Part print with two shaded views. Sizes in mm from the minimum x, y, z corner. Coordinates: 2 decimals unless noted, no trailing zeros. Loops run counter-clockwise (first coordinate to the right, second up) from the corner with the lowest first, then second, coordinate; pieces in that order, holes last.
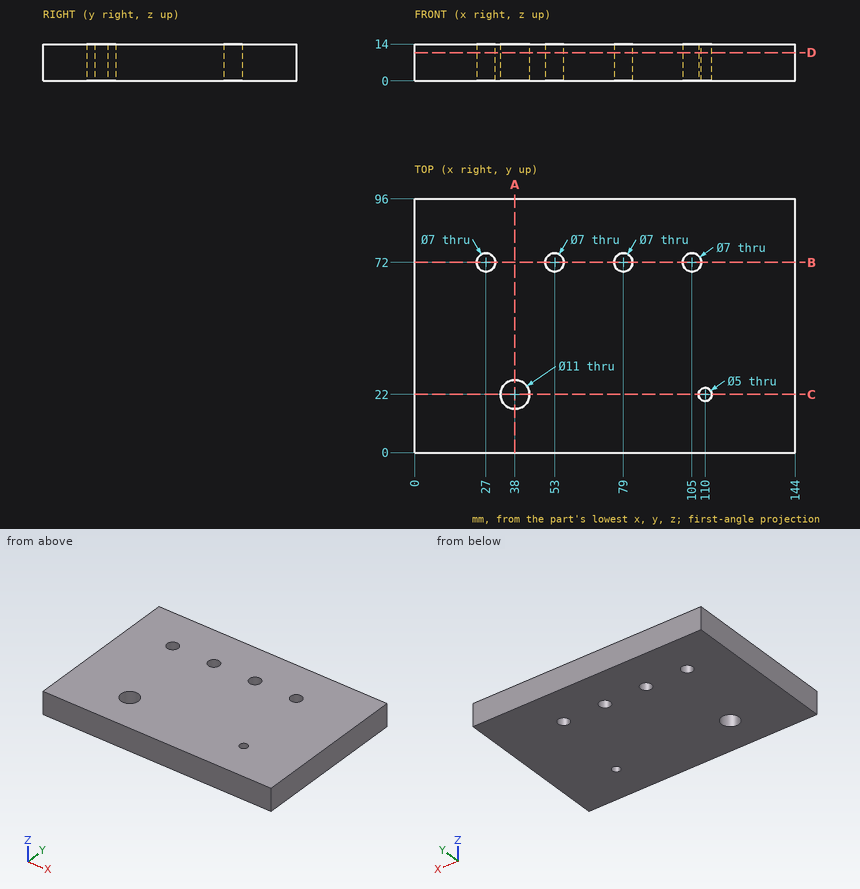
Q1. Flat gauge pins, fed straight in: P1, Ø4, axis at x = 25.5, y = 81.5, coming from the -Z side; P2, Ø3, axis at x = 110, y = 22, coming from the +Z side. Where does each tip first touch, or does it go through?
Answers:
P1: stops at z = 0
P2: passes through
Q2. Slice it at B-B (y = 72). List the corners of the cut face in (x, z).
Answers:
outline: (0, 0) - (23.5, 0) - (23.5, 14) - (0, 14) - close; (30.5, 0) - (49.5, 0) - (49.5, 14) - (30.5, 14) - close; (56.5, 0) - (75.5, 0) - (75.5, 14) - (56.5, 14) - close; (82.5, 0) - (101.5, 0) - (101.5, 14) - (82.5, 14) - close; (108.5, 0) - (144, 0) - (144, 14) - (108.5, 14) - close
Q3. Slice it at C-C (y = 22). List the corners of the cut face in (x, z).
Answers:
outline: (0, 0) - (32.5, 0) - (32.5, 14) - (0, 14) - close; (43.5, 0) - (107.5, 0) - (107.5, 14) - (43.5, 14) - close; (112.5, 0) - (144, 0) - (144, 14) - (112.5, 14) - close
Q4. Slice it at A-A (x = 38). List the corners of the cut face in (y, z).
Answers:
outline: (0, 0) - (16.5, 0) - (16.5, 14) - (0, 14) - close; (27.5, 0) - (96, 0) - (96, 14) - (27.5, 14) - close
Q5. Slice it at D-D (z = 10.75). List the corners of the cut face in (x, y), and give its area (3 significant figures).
Answers:
outline: (0, 0) - (144, 0) - (144, 96) - (0, 96) - close; hole circle Ø7 at (27, 72); hole circle Ø11 at (38, 22); hole circle Ø7 at (53, 72); hole circle Ø7 at (79, 72); hole circle Ø7 at (105, 72); hole circle Ø5 at (110, 22)
area: 13,600 mm2
Q6. Drill centre lines: line 1 (X direction, y = 22, z = 5.75); line 2 (X direction, y = 72, z = 9.5); line 3 (Y direction, x = 38, z = 3.5). Where is each one in solid material? Low to high.
Answers:
line 1: x = 0 to 32.5, 43.5 to 107.5, 112.5 to 144
line 2: x = 0 to 23.5, 30.5 to 49.5, 56.5 to 75.5, 82.5 to 101.5, 108.5 to 144
line 3: y = 0 to 16.5, 27.5 to 96
